Source: CAD feature listing. Evaluate the final solid. Frame: model axes, mm. Face numbers are marked on the shaded views. Round coordinates to 2 decimals unless told otherwise and drop trailing zeros. Write each loop counter-clockwise with the first axis right and the second up, starting at its lowest first coordinate (ties: lowest second). Pieces come first, ordered by that corner, then holes. Notation, with made-up numbers: M 67,22 L 98,22 A20 ccw 98,37 Z; hole C -1,20.25 d8. An arc over 180 degrees is marked long. Answer in a Markdown table with one row per item. Add a question column.
Item 1: Cut plane C-C on z = 18.75. Return loops of the section in (x, y), and give its area (3 significant figures).
Item 2: Cut plane A-A on z = 3. Return loops of the section in (x, y), and give its area (3 significant figures).
Item 3: Cut plane B-B on y = -40. Return loops of the section in (x, z).
Item 4: Cut plane D-D on y = -46.5. Return loops of the section in (x, z), and give its area (4 significant figures).
Item 5: Material intervals for probe 1 along Y at (x, z) = (-1.5, 11.2); probe 2 along X at (y, z) = (-28, 13.5); probe 3 along X at (y, z) = (-38, 3), sorted ascending.
Item 6: Mould query, pull axis Z, two halves, no side actions, for the marked faces 1, 2, 3 and 4. Classes: released by +Z, released by -Z, zero draft, split by the parting line, or undercut.
from build123d import *

# Parameters (mm, degrees)
F1_DEPTH = 56
F3_DEPTH = 116
F5_D     = 12
F5_DEPTH = 5
F5_TIP   = 3.6051637142


with BuildPart() as f1:
    # F0 (on Front) → F1 (new body)
    with BuildSketch(Plane.XZ):
        Polygon((-1.5, 0), (0, 0), (1.5, 0), (2, 5), (12, 5), (12.5, 0), (58, 0), (58, 25), (-58, 25), (-58, 0), (-12.5, 0), (-12, 5), (-2, 5), align=None)
    extrude(amount=F1_DEPTH)

    # F2 (on face) → F3 (cut, through all)
    with BuildSketch(Plane(origin=(-58, 0, 0), x_dir=(0, -1, 0), z_dir=(-1, 0, 0))):
        Polygon((28, 25), (20.0020753821, 25), (13, 15), (28, 15), align=None)
        Polygon((35.9979246179, 25), (28, 25), (28, 15), (43, 15), align=None)
    extrude(amount=-F3_DEPTH, mode=Mode.SUBTRACT)

    # F5
    with Locations(Plane.XY.offset(15)):
        with Locations((-1.5, -28)):
            Hole(F5_D / 2, depth=F5_DEPTH)
            with Locations((0, 0, -(F5_DEPTH + F5_TIP / 2))):  # 118° drill point
                Cone(0, F5_D / 2, F5_TIP, mode=Mode.SUBTRACT)


solid = f1.part
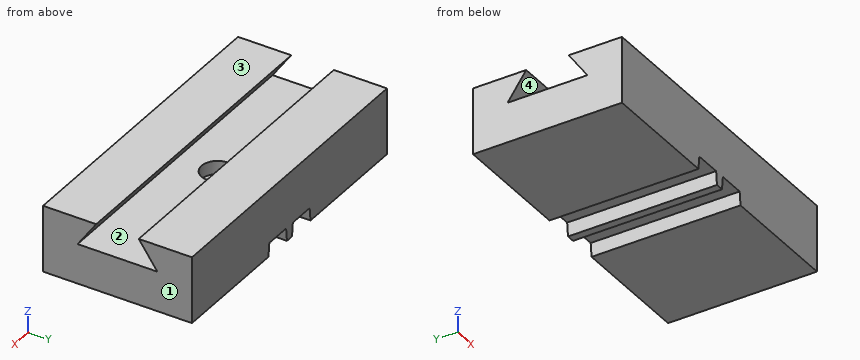
Results below:
| question | item | result |
|---|---|---|
| 1 | outline | M -58,-56 L 58,-56 L 58,-40.37 L -58,-40.37 Z; M -58,-15.63 L 58,-15.63 L 58,0 L -58,0 Z |
| 1 | area | 3,630 mm2 |
| 2 | outline | M -58,-56 L -12.2,-56 L -12.2,0 L -58,0 Z; M -1.8,-56 L 1.8,-56 L 1.8,0 L -1.8,0 Z; M 12.2,-56 L 58,-56 L 58,0 L 12.2,0 Z |
| 2 | area | 5,330 mm2 |
| 3 | outline | M -58,0 L -12.5,0 L -12,5 L -2,5 L -1.5,0 L 1.5,0 L 2,5 L 12,5 L 12.5,0 L 58,0 L 58,15 L -58,15 Z; M -58,19.28 L 58,19.28 L 58,25 L -58,25 Z |
| 4 | outline | M -58,0 L -12.5,0 L -12,5 L -2,5 L -1.5,0 L 1.5,0 L 2,5 L 12,5 L 12.5,0 L 58,0 L 58,25 L -58,25 Z |
| 4 | area | 2,795 mm2 |
| 5 | probe 1 | -56 to -34, -22 to 0 |
| 5 | probe 2 | -58 to -7.5, 4.5 to 58 |
| 5 | probe 3 | -58 to -12.2, -1.8 to 1.8, 12.2 to 58 |
| 6 | face 1 | zero draft |
| 6 | face 2 | undercut |
| 6 | face 3 | released by +Z |
| 6 | face 4 | undercut |
